Check sheet for the modelled part. Datum: model origin and axes. Units: mm. A direction names the side the tool comes from. Round coordinates to 2 decimals unless told otherwise and drop trailing zeros. Loops run counter-clockwise (first coordinate to the right, second up) from the corner with the lowest first, then second, coordinate; pieces in that order, holes last. Notation, with made-up numbers: (28.5, 77.5) -> (76.5, 77.5) arc R24 ccw to (76.5, 111.5) -> close; hole circle Ø2 at (-37.75, -14). An arc over 180 degrees is marked (long way). One line per item, written item: value. Start each with the question number.
1. Cross-section at A-A on z = 0. Record the cut outline in (x, y), then the cut area to 3 significant figures.
2. Material ranges on L1, parallel to X at y = -370, z = -1; L2, parallel to Z at x = -229, y = -155; L3, parallel to Y at x = -258, z = 0, recorded low to high.
3. Cross-section at D-D on y = -237. Record the cut outline in (x, z).
4. Cross-section at C-C on x = -159. Record the cut outline in (y, z), then the cut area to 3 significant figures.
5. Set-up check for faces 1 (the face through (-300, -141, 0)), 2 (the face through (-185, -139, 20)), 3 (the face through (-185, -141, -20)): record each of +Z, -Z, +X, -X, +Y, -Y from which the full face is reachable in a straight line by a thin tool's end or side.
6. Cross-section at B-B on y = -154.5. Record the cut outline in (x, z).
7. Go/stop test with flat-tipped pins: pin 1 (2 mm diameter, centred on y = -163.5, z = 39.5, fed in from -X); pin 2 (8 mm diameter, centred on x = -199.5, z = -2, fed in from +Y); pin 3 (4 mm diameter, centred on y = -233.5, z = 54.5, fed in from -X). Record where each tip stops, or that it passes through.
from build123d import *

# Parameters (mm, degrees)
F0_R     = 75
F1_DEPTH = 500
F3_DEPTH = 300


with BuildPart() as f1:
    # F0 (on Front) → F1 (new body)
    with BuildSketch(Plane.XZ):
        Circle(F0_R)
    extrude(amount=F1_DEPTH)

    # F2 (on Right) → F3 (join)
    with BuildSketch(Plane.YZ):
        Polygon((-100, 0), (-100, 20), (-180, 20), (-180, -20), (-100, -20), align=None)
    extrude(amount=-F3_DEPTH)


solid = f1.part
Taken from the geometry:
1. outline: (-300, -180) -> (-75, -180) -> (-75, -500) -> (75, -500) -> (75, 0) -> (-75, 0) -> (-75, -100) -> (-300, -100) -> close
1. area: 93,000 mm2
2. L1: x = -74.99 to 74.99
2. L2: z = -20 to 20
2. L3: y = -180 to -100
3. outline: circle Ø150 at (0, 0)
4. outline: (-180, -20) -> (-100, -20) -> (-100, 20) -> (-180, 20) -> close
4. area: 3,200 mm2
5. face 1: +Z, -Z, -X, +Y, -Y
5. face 2: +Z, -X, +Y, -Y
5. face 3: -Z, -X, +Y, -Y
6. outline: (-300, -20) -> (-72.28, -20) arc R75 ccw (long way) to (-72.28, 20) -> (-300, 20) -> close
7. pin 1: stops at x = -64.36
7. pin 2: stops at y = -100
7. pin 3: stops at x = -53.56
